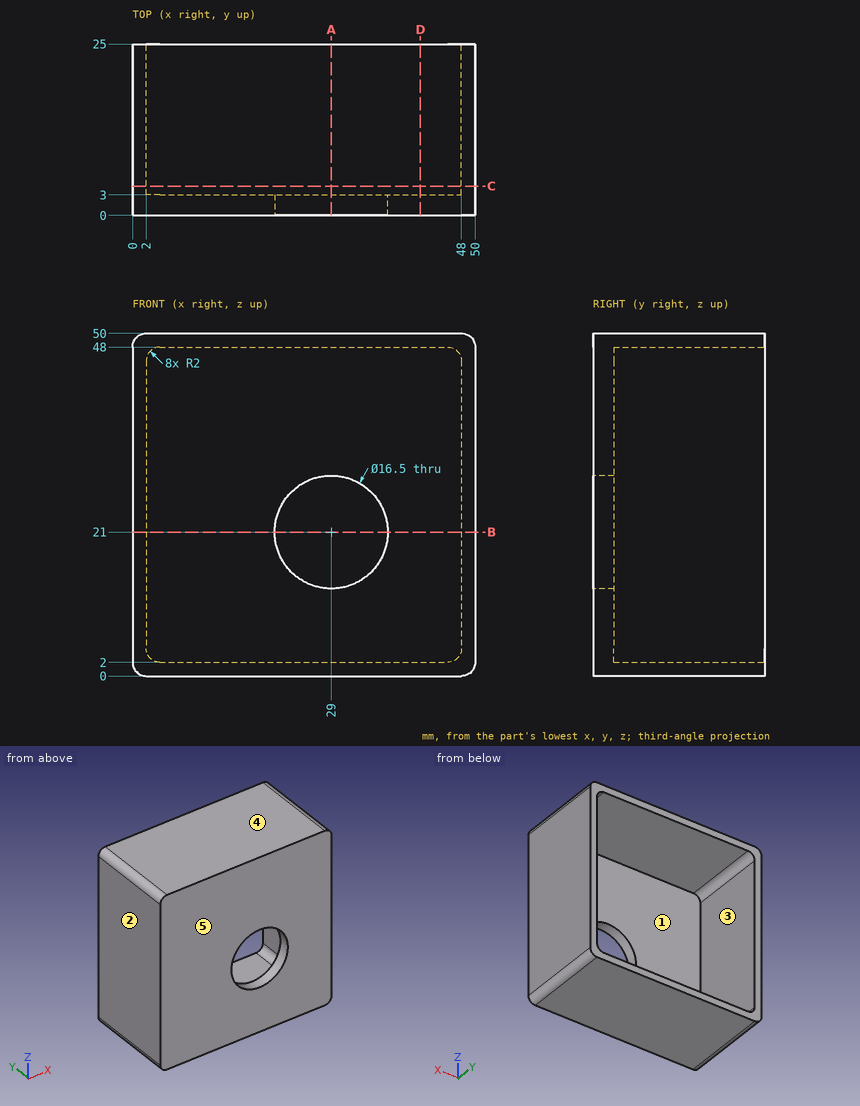
Input: dimensioned drawing with shaded views. Units: mm. Origin: part minimum x, y, z. A direction names the side the tool comes from. Give positions to 0.01 mm unless a question says otherwise; leave off trailing zeros. Write each loop counter-clockwise with the first axis right and the second up, starting at its lowest first coordinate (ties: lowest second). Pieces come first, ordered by that corner, then holes. Notation, with made-up numbers: M -4,-35 L 35,-35 A19 ccw 35,-28 Z; hole C -11.75,2 d8. An arc over 180 degrees is marked long. Write item = value, one per line. Start each with the question number.
1) Cut plane D-D on x = 42. Return the cut outline in (y, z).
2) Draft query along Z for the marked faces 3, 4 and 5. Return one class per face: +Z half, -Z half, draft (parallel to the pull), parting line (faces both ways), or undercut.
3) Reachability of the marked faces 1 and 2 from +Z, -Z, +X, -X, +Y, -Y: full face, straight path, thin tool, end or side. Return the list, or none.
4) Material intervals for line 1 along Z through (x, y) = (37.5, 12); line 2 along X through (y, z) = (1.55, 21), sorted ascending. Write a range as [from, to].
5) Cut plane A-A on x = 29. Return the cut outline in (y, z).
6) Cut plane B-B on z = 21. Return the cut outline in (x, y).
7) Cut plane C-C on y = 4.25. Return the cut outline in (x, z).
8) First-contact query: pin 1 Ø12 at (x, z) = (27, 27.5) entering from +Y. Flat tip, straight axial feed; report the tip coordinate or a pass-through.
Solved:
q1.outline = M 0,0 L 25,0 L 25,2 L 3,2 L 3,48 L 25,48 L 25,50 L 0,50 Z
q2.face_3 = undercut
q2.face_4 = +Z half
q2.face_5 = draft
q3.face_1 = +Y
q3.face_2 = +Z, -Z, -X, +Y, -Y
q4.line_1 = [0, 2], [48, 50]
q4.line_2 = [0, 20.75], [37.25, 50]
q5.outline = M 0,0 L 25,0 L 25,2 L 3,2 L 3,12.75 L 0,12.75 Z; M 0,29.25 L 3,29.25 L 3,48 L 25,48 L 25,50 L 0,50 Z
q6.outline = M 0,0 L 20.75,0 L 20.75,3 L 2,3 L 2,25 L 0,25 Z; M 37.25,0 L 50,0 L 50,25 L 48,25 L 48,3 L 37.25,3 Z
q7.outline = M 0,2 A2 ccw 2,0 L 48,0 A2 ccw 50,2 L 50,48 A2 ccw 48,50 L 2,50 A2 ccw 0,48 Z; hole M 2,4 A2 ccw 4,2 L 46,2 A2 ccw 48,4 L 48,46 A2 ccw 46,48 L 4,48 A2 ccw 2,46 Z
q8.pin_1 = 3
